Could you check a few things on this model? Use its own coordinates, in mm. A direction names the side the tool comes from. Round coordinates to 2 decimals unless told otherwise and drop trailing zeros. Order: outer loops, then holes, each group sorted by start corner. A loop starts at its lowest first (then second) coordinate and runs counter-clockwise, first axis right, second up.
```python
from build123d import *

# Parameters (mm, degrees)
SKETCH1_R           = 84
SKETCH1_R_2         = 79
BOSS_EXTRUDE1_DEPTH = 25
SKETCH2_R           = 84
BOSS_EXTRUDE2_DEPTH = 5
SKETCH3_R           = 81
SKETCH3_R_2         = 77
BOSS_EXTRUDE3_DEPTH = 80
FILLET1_R           = 10
CUT_EXTRUDE1_REACH  = 148.072
SKETCH4_W           = 14
SKETCH4_H           = 7
CUT_EXTRUDE2_REACH  = 145.22
SKETCH5_W           = 10
SKETCH5_H           = 16
FILLET2_R           = 1


with BuildPart() as part:
    # Sketch1 → Boss-Extrude1 (new body)
    with BuildSketch(Plane(origin=(0, 0, 0), x_dir=(1, 0, 0), z_dir=(0, 1, 0))):
        with Locations(Location((0, 0, 0), (0, 0, 270))):
            Circle(SKETCH1_R)
        with Locations(Location((0, 0, 0), (0, 0, 270))):
            Circle(SKETCH1_R_2, mode=Mode.SUBTRACT)
    extrude(amount=BOSS_EXTRUDE1_DEPTH)

    # Sketch2 → Boss-Extrude2 (add)
    with BuildSketch(Plane(origin=(0, 25, 0), x_dir=(1, 0, 0), z_dir=(0, 1, 0))):
        with Locations(Location((0, 0, 0), (0, 0, 270))):
            Circle(SKETCH2_R)
    extrude(amount=BOSS_EXTRUDE2_DEPTH)

    # Sketch3 → Boss-Extrude3 (add)
    with BuildSketch(Plane(origin=(0, 30, 0), x_dir=(1, 0, 0), z_dir=(0, 1, 0))):
        with Locations(Location((0, 0, 0), (0, 0, 270))):
            Circle(SKETCH3_R)
        with Locations(Location((0, 0, 0), (0, 0, 270))):
            Circle(SKETCH3_R_2, mode=Mode.SUBTRACT)
    extrude(amount=BOSS_EXTRUDE3_DEPTH)

    # Fillet1
    fillet1_edges = [part.edges().sort_by_distance(p)[0] for p in [
        (0, 25, -79),
        (0, 30, -77),
    ]]
    fillet(fillet1_edges, radius=FILLET1_R)

    # Sketch4 → Cut-Extrude1 (cut, up to next)
    with BuildSketch(Plane.XZ.offset(-25), mode=Mode.PRIVATE) as cut_extrude1_sk1:
        Rectangle(SKETCH4_W, SKETCH4_H)
    cut_extrude1_tool1 = extrude(cut_extrude1_sk1.sketch, amount=-CUT_EXTRUDE1_REACH, mode=Mode.PRIVATE) & part.part
    add(cut_extrude1_tool1.solids().sort_by_distance((0, 25, 0))[0], mode=Mode.SUBTRACT)

    # Sketch5 → Cut-Extrude2 (cut, up to next)
    with BuildSketch(Plane(origin=(0, 30, 0), x_dir=(1, 0, 0), z_dir=(0, 1, 0)), mode=Mode.PRIVATE) as cut_extrude2_sk1:
        with Locations((-50, 0)):
            Rectangle(SKETCH5_W, SKETCH5_H)
    cut_extrude2_tool1 = extrude(cut_extrude2_sk1.sketch, amount=-CUT_EXTRUDE2_REACH, mode=Mode.PRIVATE) & part.part
    add(cut_extrude2_tool1.solids().sort_by_distance((-50, 30, 0))[0], mode=Mode.SUBTRACT)

    # Fillet2
    fillet2_edges = [part.edges().sort_by_distance(p)[0] for p in [
        (0, 30, 3.5),
        (7, 30, 0),
        (0, 30, -3.5),
        (-7, 30, 0),
        (0, 25, 3.5),
        (-7, 25, 0),
        (0, 25, -3.5),
        (7, 25, 0),
        (-55, 30, 0),
        (-50, 30, 8),
        (-45, 30, 0),
        (-50, 30, -8),
        (-50, 25, 8),
        (-55, 25, 0),
        (-50, 25, -8),
        (-45, 25, 0),
    ]]
    fillet(fillet2_edges, radius=FILLET2_R)


solid = part.part
```
Q1. I need wall thicknesses on L1, parallel to X at y = 67, z = 0; L2, parallel to X at y = 3.5, z = 0; L3, parallel to Y at x = -23.5, z = -26.5. Which ranges of each line are inside material? Lowest first, please.
Q2. We'd pull the mould along Z, two halves only. Please class faces 1 (the flat face through (-72, 110, 30)), 2 (the flat face through (-14, 30, -1)), 3 (the cylindrical face through (25.23, 14.79, 80.12)), 4 (the cylindrical face through (-75.17, 74.51, -16.69)): released by +Z, released by -Z, zero draft, split by the parting line, or undercut.
Q3. Imagine slicing it at A-A, the plane x = 0. Please give me the cut outline in (y, z).
Q4. Imagine slicing it at C-C, the plane z = 0. State how many separate pieces and enclosed holes the cut face has, then the cut area to 3 significant figures.
Q5. Imagine slicing it at B-B, the plane y = 44. Please give me the cut outline in (x, z), then the cut area to 3 significant figures.
Q6. For P1, Ø5, axis at x = -12.5, z = 44, coming from the +Y side; P2, Ø1.5, axis at x = 28.5, y = 88, coming from the -Z side; P3, Ø3.5, axis at y = 27.5, z = 2.5, coming from the +X side, each with a flat end and sliding along its axis, tell me the tip position at first contact or that it passes through.
Q7. For faces 5 (the cylindrical face through (23.73, 7.4, 75.35)), 6 (the flat face through (-56, 0, -56)), 7 (the flat face through (44, 30, -69)), which set-ups out of +Z, -Z, +X, -X, +Y, -Y let a thin tool reach every point of the face, with its end or its side?
Filled in:
1. L1: x = -81 to -77, 77 to 81
1. L2: x = -84 to -79, 79 to 84
1. L3: y = 25 to 30
2. face 1: zero draft
2. face 2: undercut
2. face 3: split by the parting line
2. face 4: undercut
3. outline: (0, -84) - (30, -84) - (30, -81) - (110, -81) - (110, -77) - (40, -77) arc R10 cw to (30, -67) - (30, -4.5) arc R1 ccw to (29, -3.5) - (26, -3.5) arc R1 ccw to (25, -4.5) - (25, -69) arc R10 cw to (15, -79) - (0, -79) - close; (0, 79) - (15, 79) arc R10 cw to (25, 69) - (25, 4.5) arc R1 ccw to (26, 3.5) - (29, 3.5) arc R1 ccw to (30, 4.5) - (30, 67) arc R10 cw to (40, 77) - (110, 77) - (110, 81) - (30, 81) - (30, 84) - (0, 84) - close
4. separate pieces: 3
4. enclosed holes: 0
4. area: 1,690 mm2
5. outline: circle Ø162 at (0, 0); hole circle Ø154 at (0, 0)
5. area: 1,990 mm2
6. P1: stops at y = 30
6. P2: stops at z = -76.1
6. P3: stops at x = 84
7. face 5: -Y
7. face 6: +Z, -Z, +X, -X, -Y
7. face 7: +Y
